```python
from build123d import *

# Parameters (mm, degrees)
SKETCH1_W               = 40
SKETCH1_H               = 35
BOSS_EXTRUDE1_DEPTH     = 8
CUT_EXTRUDE1_DEPTH      = 1
CUT_EXTRUDE1_DEPTH_BACK = 41
FILLET1_R               = 2
SKETCH4_W               = 35
SKETCH4_H               = 2
BOSS_EXTRUDE2_DEPTH     = 10
SKETCH5_W               = 35
SKETCH5_H               = 2
BOSS_EXTRUDE3_DEPTH     = 12
SKETCH6_R               = 1.6
CUT_EXTRUDE2_DEPTH      = 10
SKETCH7_W               = 8
SKETCH7_H               = 6.5
SKETCH7_H_2             = 8
CUT_EXTRUDE3_DEPTH      = 3
SKETCH8_W               = 20
SKETCH8_H               = 2
CUT_EXTRUDE5_DEPTH      = 36
FILLET2_R               = 2
SKETCH10_R              = 1.6
CUT_EXTRUDE6_DEPTH      = 3
BOSS_EXTRUDE4_DEPTH     = 2


with BuildPart() as part:
    # Sketch1 → Boss-Extrude1 (new body)
    with BuildSketch(Plane(origin=(0, 0, 0), x_dir=(1, 0, 0), z_dir=(0, 1, 0))):
        Rectangle(SKETCH1_W, SKETCH1_H)
    extrude(amount=-BOSS_EXTRUDE1_DEPTH)

    # Sketch2 → Cut-Extrude1 (cut, two sides)
    with BuildSketch(Plane(origin=(20, 0, 0), x_dir=(0, 0, -1), z_dir=(1, 0, 0))) as cut_extrude1_sk:
        Polygon((-12.5, -5), (-17.5, -8), (0, -8), (0, -5), align=None)
        Polygon((0, -5), (0, -8), (17.5, -8), (12.5, -5), align=None)
    extrude(amount=CUT_EXTRUDE1_DEPTH, mode=Mode.SUBTRACT)
    extrude(cut_extrude1_sk.sketch, amount=-CUT_EXTRUDE1_DEPTH_BACK, mode=Mode.SUBTRACT)

    # Fillet1
    fillet1_edges = [part.edges().sort_by_distance(p)[0] for p in [
        (0, -8, -17.5),
        (0, -5, 12.5),
        (0, -5, -12.5),
        (0, -8, 17.5),
    ]]
    fillet(fillet1_edges, radius=FILLET1_R)

    # Sketch4 → Boss-Extrude2 (add)
    with BuildSketch(Plane.ZY.offset(20)):
        with Locations((0, -1)):
            Rectangle(SKETCH4_W, SKETCH4_H)
    extrude(amount=BOSS_EXTRUDE2_DEPTH)

    # Sketch5 → Boss-Extrude3 (add)
    with BuildSketch(Plane(origin=(20, 0, 0), x_dir=(0, 0, -1), z_dir=(1, 0, 0))):
        with Locations((0, -1)):
            Rectangle(SKETCH5_W, SKETCH5_H)
    extrude(amount=BOSS_EXTRUDE3_DEPTH)

    # Sketch6 → Cut-Extrude2 (cut)
    with BuildSketch(Plane.XZ.offset(2)):
        with Locations((-25, 15)):
            Circle(SKETCH6_R)
        with Locations((-25, -15)):
            Circle(SKETCH6_R)
    extrude(amount=-CUT_EXTRUDE2_DEPTH, mode=Mode.SUBTRACT)

    # Sketch7 → Cut-Extrude3 (cut)
    with BuildSketch(Plane(origin=(0, 0, 0), x_dir=(1, 0, 0), z_dir=(0, 1, 0))):
        with Locations((-14.5, 14.25)):
            Rectangle(SKETCH7_W, SKETCH7_H)
        with Locations((-14.5, -15)):
            Rectangle(SKETCH7_W, SKETCH7_H_2)
    extrude(amount=-CUT_EXTRUDE3_DEPTH, mode=Mode.SUBTRACT)

    # Sketch8 → Cut-Extrude5 (cut, through all)
    with BuildSketch(Plane.XY.offset(17.5)):
        with Locations((4, -1)):
            Rectangle(SKETCH8_W, SKETCH8_H)
    extrude(amount=-CUT_EXTRUDE5_DEPTH, mode=Mode.SUBTRACT)

    # Fillet2
    fillet2_edges = [part.edges().sort_by_distance(p)[0] for p in [
        (-10.5, -1.5, -11),
        (-18.5, -1.5, -11),
        (-18.5, -1.5, 11),
        (-10.5, -1.5, 11),
    ]]
    fillet(fillet2_edges, radius=FILLET2_R)

    # Sketch10 → Cut-Extrude6 (cut, through all)
    with BuildSketch(Plane.XZ.offset(2)):
        with Locations((28.5, 15.5)):
            Circle(SKETCH10_R)
        with Locations((28.5, -15.5)):
            Circle(SKETCH10_R)
    extrude(amount=-CUT_EXTRUDE6_DEPTH, mode=Mode.SUBTRACT)

    # Sketch10<4> → Boss-Extrude4 (add)
    with BuildSketch(Plane.XZ.offset(2)):
        with BuildLine():
            ThreePointArc((31.964101615, 17.5), (28.5, 19.5), (25.035898385, 17.5))
            Line((25.035898385, 17.5), (31.964101615, 17.5))
        make_face()
        with BuildLine():
            Line((32, 17.436491673), (32, 13.563508327))
            ThreePointArc((32, 13.563508327), (32.372983346, 14.5), (32.5, 15.5))
            ThreePointArc((32.5, 15.5), (32.372983346, 16.5), (32, 17.436491673))
        make_face()
        with BuildLine():
            Line((31.964101615, -17.5), (25.035898385, -17.5))
            ThreePointArc((25.035898385, -17.5), (28.5, -19.5), (31.964101615, -17.5))
        make_face()
        with BuildLine():
            ThreePointArc((32.5, -15.5), (32.372983346, -14.5), (32, -13.563508327))
            Line((32, -13.563508327), (32, -17.436491673))
            ThreePointArc((32, -17.436491673), (32.372983346, -16.5), (32.5, -15.5))
        make_face()
        with BuildLine():
            ThreePointArc((32.5, 15.5), (32.372983346, 14.5), (32, 13.563508327))
            Line((32, 13.563508327), (32, -13.563508327))
            ThreePointArc((32, -13.563508327), (32.372983346, -14.5), (32.5, -15.5))
            Line((32.5, -15.5), (32.5, 15.5))
        make_face()
    extrude(amount=-BOSS_EXTRUDE4_DEPTH)


solid = part.part
```
Work out the finished part from the listing and answer in its coordinate system (mm). A direction names the side the tool comes from. Round coordinates to 2 decimals unless told otherwise and drop trailing zeros. Order: outer loops, then holes, each group sorted by start corner. A loop starts at its lowest first (then second) coordinate and runs counter-clockwise, first axis right, second up.
Q1. Given pin 1 Ø3 at (x, z) = (-25.5, 6) entering from -Y; pin 2 Ø1.3 at (x, y) = (3, -1) entering from +Z; pin 3 Ø2.5 at (x, y) = (-14, -2) entering from -Z; pin 4 Ø8 at (x, z) = (7.5, -8.5) entering from +Y, each flat-ended and moving along its own axis, determine where each tip first touches the part or whether it passes through.
Solution:
pin 1: stops at y = -2
pin 2: passes through
pin 3: stops at z = -17.5
pin 4: stops at y = -2
Q2. A cutting plane is placed at A-A, the plane y = -1.25. Count the separate pieces of the cut face and the enclosed holes in it, then the cut area to 3 significant figures.
Solution:
separate pieces: 2
enclosed holes: 4
area: 1,370 mm2
Q3. A tool of negligible diameter and unlimited length cuts with its end or side. For faces 4 (the cylindrical face through (-17.93, -1.52, 11.6)), 5 (the flat face through (0.28, -5.74, -13.73)), 6 (the flat face through (-18.5, -1, -15)), 7 (the flat face through (14, -1, 0)), from which of +Z, -Z, +X, -X, +Y, -Y can it reach the whole face along a straight path? Write none if from no direction.
Solution:
face 4: +Z, +Y
face 5: +X, -X, -Y
face 6: -Z, +Y
face 7: +Z, -Z, +Y
Q4. Find the intervals of material crossed by line 1 along Z through (x, y) = (-25, -1.45); line 2 along Z through (x, y) = (28.5, -0.5); line 3 along X through (y, z) = (-0.75, -0.5), in increasing order.
Solution:
line 1: z = -17.5 to -16.6, -13.4 to 13.4, 16.6 to 17.5
line 2: z = -19.5 to -17.1, -13.9 to 13.9, 17.1 to 19.5
line 3: x = -30 to -6, 14 to 32.5
Q5. The mould has two halves that part along X. Classify faces 1 (the flat face through (20, -4, 0)), 2 (the flat face through (26, -2, 0)), 3 (the cylindrical face through (-11.1, -1.52, -11.57)): pulls with the +X half, pulls with the -X half, needs draft (parallel to the pull), parting line crosses it, or undercut.
Solution:
face 1: pulls with the +X half
face 2: needs draft
face 3: undercut
Q6. A cutting plane is placed at C-C, the plane z = 7. Determine the outline of the cut face in (x, y), then the cut area to 3 significant figures.
Solution:
outline: (-30, -2) - (-20, -2) - (-20, -5) - (20, -5) - (20, -2) - (32.5, -2) - (32.5, 0) - (14, 0) - (14, -2) - (-6, -2) - (-6, 0) - (-30, 0) - close
area: 205 mm2
Q7. A cutting plane is placed at D-D, the plane x = 9.5. Determine the outline of the cut face in (y, z), then the cut area to 3 significant figures.
Solution:
outline: (-6.18, -14.47) arc R2 ccw to (-4.47, -17.5) - (-2, -17.5) - (-2, 17.5) - (-4.47, 17.5) arc R2 ccw to (-6.18, 14.47) - (-5.29, 12.98) arc R2 cw to (-5, 11.95) - (-5, -11.95) arc R2 cw to (-5.29, -12.98) - close
area: 114 mm2
Q8. A cutting plane is placed at B-B, the plane x = 28.5. Determine the outline of the cut face in (y, z).
Solution:
outline: (-2, -19.5) - (0, -19.5) - (0, -17.1) - (-2, -17.1) - close; (-2, -13.9) - (0, -13.9) - (0, 13.9) - (-2, 13.9) - close; (-2, 17.1) - (0, 17.1) - (0, 19.5) - (-2, 19.5) - close
